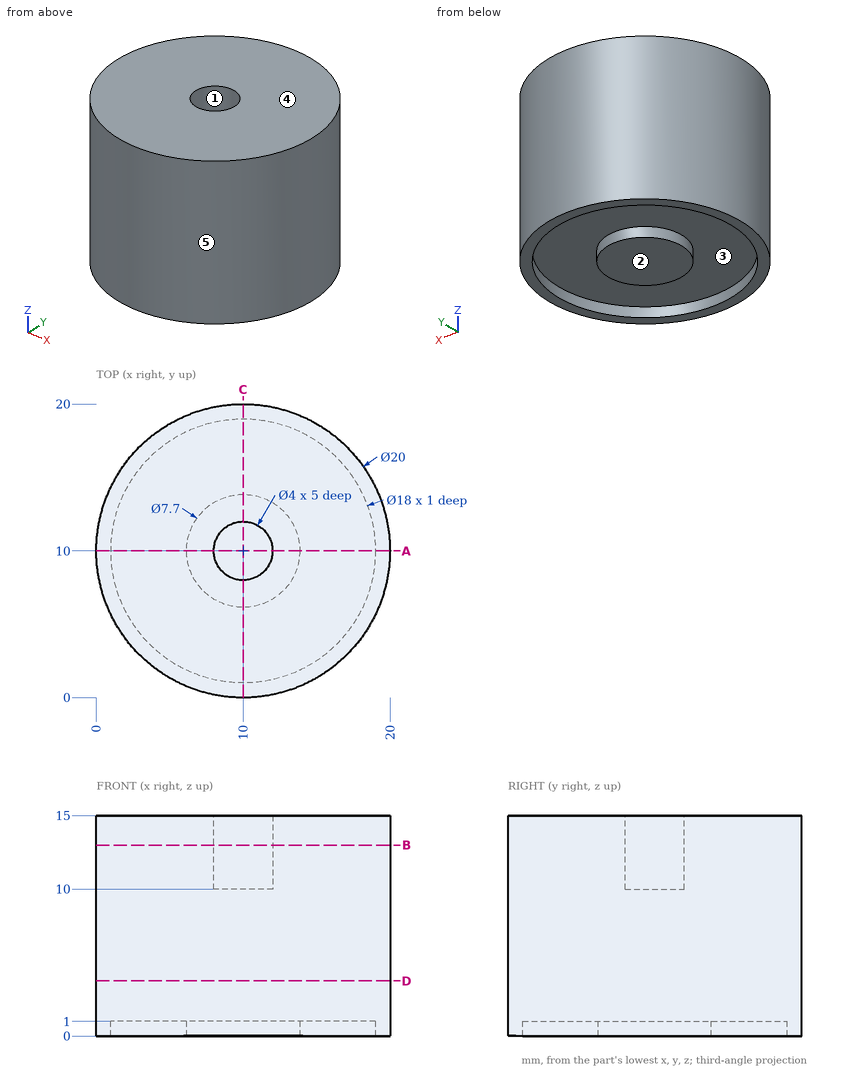
Geometry: see drawing. Coordinates: mm, zero at the bounding-box minimum. A direction names the side the tool comes from. Round coordinates to 2 decimals unless told otherwise and drop trailing zeros. Loops run counter-clockwise (first coordinate to the right, second up) from the corner with the lowest first, then second, coordinate; pieces in that order, holes last. Notation, with made-up numbers: M 60.25,-3.75 L 82.25,-3.75 A28 ccw 82.25,31.25 Z; hole C 64,-6.5 d8. An arc over 180 degrees is marked long. Use a Markdown table: item, result. Add a question column.
1. Section query B-B on z = 13. Return the cut outline in (x, y), then the cut area to 3 significant figures.
2. Line query: line 1 (X direction, y = 10, z = 0.45); line 2 (X direction, y = 10, z = 11.65). Output: solid intervals per line, ascending.
3. Section query A-A on y = 10. Return the cut outline in (x, z), then the cut area to 3 significant figures.
4. Mould query, pull axis Y, two halves, no side actions, for the marked faces 3, 4 and 5. Classes: pulls with the +Y half, pulls with the -Y half, needs draft (parallel to the pull), parting line crosses it, or undercut.
5. Section query D-D on z = 3.75. Return the cut outline in (x, y).
6. Contact query for flat-ended pins moving along their axis: P1, Ø2, axis at x = 16.5, z = 3.5, coming from the +Y side; P2, Ø2, axis at x = 4, z = 5.5, coming from the -Y side; P3, Ø1, axis at y = 13, z = 7, coming from the -X side. Output: stop coordinate, or through.
7. Reachability of the marked faces 1 and 2 from +Z, -Z, +X, -X, +Y, -Y: full face, straight path, thin tool, end or side. Return the list, or none.
Reported:
| question | item | result |
|---|---|---|
| 1 | outline | C 10,10 d20; hole C 10,10 d4 |
| 1 | area | 302 mm² |
| 2 | line 1 | x = 0 to 1, 6.15 to 13.85, 19 to 20 |
| 2 | line 2 | x = 0 to 8, 12 to 20 |
| 3 | outline | M 0,0 L 1,0 L 1,1 L 6.15,1 L 6.15,0 L 13.85,0 L 13.85,1 L 19,1 L 19,0 L 20,0 L 20,15 L 12,15 L 12,10 L 8,10 L 8,15 L 0,15 Z |
| 3 | area | 270 mm² |
| 4 | face 3 | undercut |
| 4 | face 4 | needs draft |
| 4 | face 5 | parting line crosses it |
| 5 | outline | C 10,10 d20 |
| 6 | P1 | stops at y = 18.35 |
| 6 | P2 | stops at y = 1.34 |
| 6 | P3 | stops at x = 0.32 |
| 7 | face 1 | +Z |
| 7 | face 2 | -Z, +X, -X, +Y, -Y |
